from build123d import *

# Parameters (mm, degrees)
SKETCH1_R           = 1.5
BOSS_EXTRUDE1_DEPTH = 1.6
SKETCH2_W           = 121
SKETCH2_H           = 78
BOSS_EXTRUDE2_DEPTH = 7


with BuildPart() as part:
    # Sketch1 → Boss-Extrude1 (new body)
    with BuildSketch(Plane(origin=(0, 0, 0), x_dir=(1, 0, 0), z_dir=(0, 1, 0))):
        Polygon((-166.842260972, 58.195002586), (-166.842260972, -19.804997414), (-166.842260972, -25.804997414), (-160.842260972, -25.804997414), (-160.842260972, -19.804997414), (-51.842260972, -19.804997414), (-51.842260972, -25.804997414), (-45.842260972, -25.804997414), (-45.842260972, -19.804997414), (-45.842260972, 58.195002586), (-45.842260972, 64.195002586), (-51.842260972, 64.195002586), (-51.842260972, 58.195002586), (-160.842260972, 58.195002586), (-160.842260972, 64.195002586), (-166.842260972, 64.195002586), align=None)
        with Locations(Location((-48.842260972, -22.804997414, 0), (0, 0, 270))):
            Circle(SKETCH1_R, mode=Mode.SUBTRACT)
        with Locations(Location((-163.842260972, -22.804997414, 0), (0, 0, 270))):
            Circle(SKETCH1_R, mode=Mode.SUBTRACT)
        with Locations(Location((-48.842260972, 61.195002586, 0), (0, 0, 90))):
            Circle(SKETCH1_R, mode=Mode.SUBTRACT)
        with Locations(Location((-163.842260972, 61.195002586, 0), (0, 0, 90))):
            Circle(SKETCH1_R, mode=Mode.SUBTRACT)
    extrude(amount=BOSS_EXTRUDE1_DEPTH)

    # Sketch2 → Boss-Extrude2 (add)
    with BuildSketch(Plane(origin=(0, 1.6, 0), x_dir=(1, 0, 0), z_dir=(0, 1, 0))):
        with Locations((-106.342260972, 19.195002586)):
            Rectangle(SKETCH2_W, SKETCH2_H)
    extrude(amount=BOSS_EXTRUDE2_DEPTH)


solid = part.part
Verification items for the finished model (mm, model axes). A direction names the side the tool comes from. Round coordinates to 2 decimals unless told otherwise and drop trailing zeros. Write each loop counter-clockwise with the first axis right and the second up, starting at its lowest first coordinate (ties: lowest second). Pieces come first, ordered by that corner, then holes.
(1) Access from +Z, -Z, +X, -X, +Y, -Y to the whole of each face (thin tool, end or side, straight path). Record for faces 3 (the flat face through (-50, 1.6, 21)), 4 (the flat face through (-165, 1.6, -63)), 5 (the cylindrical face through (-165.33, 0.79, -61)).
Returned:
face 3: +Z, +X, -X, +Y
face 4: -Z, +X, -X, +Y
face 5: +Y, -Y
(2) Mould release check, pull along Z, two halves, no side actions. Record for faces 1 (the flat face through (-166.842, 4, -19)), 2 (the cylindrical face through (-47.355, 0.789, 22.61)): pulls with the +Z half, pulls with the -Z half, needs draft (parallel to the pull), parting line crosses it, or undercut.
Returned:
face 1: needs draft
face 2: undercut
(3) Section check B-B (y = 3). Enter the section's corners in (x, z) (3 decimals).
Returned:
outline: (-166.842, -58.195) - (-45.842, -58.195) - (-45.842, 19.805) - (-166.842, 19.805) - close
(4) Depth check by flat-ended pin: pin 1 Ø3 at (x, z) = (-164, 23) entering from +Y; pin 2 Ø5 at (x, y) = (-106.5, 5.5) entering from -Z (3 decimals); pin 3 Ø2 at (x, y) = (-91, 2) entering from +Z (3 decimals); pin 4 Ø1.8 at (x, z) = (-48.84, 22.8) entering from -Y. Enter the tip coordinate at first touch or a pass-through.
Returned:
pin 1: stops at y = 1.6
pin 2: stops at z = -58.195
pin 3: stops at z = 19.805
pin 4: passes through
(5) Material ranges on line 1 (X direction, y = 1, z = 22); line 2 (Z direction, x = -109, y = 8) (3 decimals), recorded low to high.
Returned:
line 1: x = -166.84 to -165.11, -162.58 to -160.84, -51.84 to -50.11, -47.58 to -45.84
line 2: z = -58.195 to 19.805
(6) Section check A-A (x = -119.5). Enter the section's corners in (y, z) (3 decimals).
Returned:
outline: (0, -58.195) - (8.6, -58.195) - (8.6, 19.805) - (0, 19.805) - close
